```python
from build123d import *

# Parameters (mm, degrees)
PAD_DEPTH       = 10
POCKET_DEPTH    = 10.001
SKETCH002_W     = 1
SKETCH002_H     = 10
PAD001_DEPTH    = 7
SKETCH003_R     = 2
POCKET001_DEPTH = 5
FILLET_R        = 1


with BuildPart() as part:
    # Sketch → Pad (new body)
    with BuildSketch(Plane.XZ):
        with BuildLine():
            ThreePointArc((3.5, 3.5), (0, 6), (-3.5, 3.5))
            Line((-3.5, 3.5), (-3.5, 0))
            Line((-3.5, 0), (3.5, 0))
            Line((3.5, 0), (3.5, 3.5))
        make_face()
    extrude(amount=PAD_DEPTH)

    # Sketch001 (on Face6 of Pad) → Pocket (cut, through all)
    with BuildSketch(Plane.XZ.offset(10)):
        with BuildLine():
            ThreePointArc((2.5, 2.5), (0, 5), (-2.5, 2.5))
            Line((-2.5, 2.5), (-2.5, 0))
            Line((-2.5, 0), (2.5, 0))
            Line((2.5, 0), (2.5, 2.5))
        make_face()
    extrude(amount=-POCKET_DEPTH, mode=Mode.SUBTRACT)

    # Sketch002 (on Face3 of Pocket) → Pad001 (join)
    with BuildSketch(Plane(origin=(-3.5, 0, 0), x_dir=(0, 0, -1), z_dir=(-1, 0, 0))):
        with Locations((-0.5, 5)):
            Rectangle(SKETCH002_W, SKETCH002_H)
    extrude(amount=PAD001_DEPTH)

    # Sketch003 (on Face7 of Pad001) → Pocket001 (cut)
    with BuildSketch(Plane(origin=(0, 0, 1), x_dir=(-1, 0, 0), z_dir=(0, 0, 1))):
        with Locations((7, 5)):
            Circle(SKETCH003_R)
    extrude(amount=-POCKET001_DEPTH, mode=Mode.SUBTRACT)

    # Fillet
    fillet_edges = [part.edges().sort_by_distance(p)[0] for p in [
        (-10.5, -10, 0.5),
        (-10.5, 0, 0.5),
    ]]
    fillet(fillet_edges, radius=FILLET_R)


solid = part.part
```
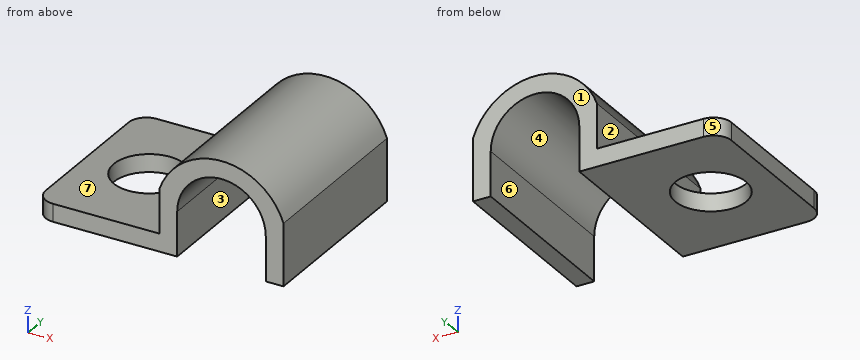
Source: CAD feature listing. Evaluate the final solid. Frame: model axes, mm. Face numbers are marked on the shaded views. A direction names the side the tool comes from. Coordinates: 2 decimals unless noted, no trailing zeros. Write each loop counter-clockwise with the first axis right and the second up, starting at its lowest first coordinate (ties: lowest second). Pieces come first, ordered by that corner, then holes. Notation, with made-up numbers: (86.25, 60.25) - (104.25, 60.25) arc R27 ccw to (104.25, 84.25) - close; hole circle Ø10 at (64, 77). An arc over 180 degrees is marked (long way). Answer as a JSON object with one key per item and string values.
Q1. Set-up query: the marked faces 1, 2 and 3. Return all of +Z, -Z, +X, -X, +Y, -Y with unobstructed straight access to the full face (end or side cutting, diameter ignored); none if empty.
Ans:
{"face 1": "+Z, -Z, +X, -X, +Y", "face 2": "+Z, -X, +Y, -Y", "face 3": "-Z, +Y, -Y"}
Q2. Section query B-B, the plane z = 1.8. Output: boundary loops of the cut face in (x, y), plus the area to 3 significant figures.
Ans:
{"outline": "(-3.5, -10) - (-2.5, -10) - (-2.5, 0) - (-3.5, 0) - close; (2.5, -10) - (3.5, -10) - (3.5, 0) - (2.5, 0) - close", "area": "20.0 mm2"}
Q3. Material intervals for line 1 (X direction, y = -5, z = 0.85); line 2 (X direction, y = -6.5, z = 2.3); line 3 (X direction, y = -5.5, z = 0.55), sorted ascending. Write a range as [from, to].
Ans:
{"line 1": "x = [-10.5, -9], [-5, -2.5], [2.5, 3.5]", "line 2": "x = [-3.5, -2.5], [2.5, 3.5]", "line 3": "x = [-10.5, -8.94], [-5.06, -2.5], [2.5, 3.5]"}
Q4. Section query A-A, the plane x = -7. Output: boundary loops of the cut face in (y, z), plus the area to 3 significant figures.
Ans:
{"outline": "(-10, 0) - (-7, 0) - (-7, 1) - (-10, 1) - close; (-3, 0) - (0, 0) - (0, 1) - (-3, 1) - close", "area": "6.00 mm2"}
Q5. First-contact query: pin 1 Ø1.5 at (x, z) = (-7.5, 2.5) entering from -Y; pin 2 Ø5.5 at (x, y) = (-8.5, -3) entering from +Z; pin 3 Ø1 at (y, z) = (-4.5, 5) entering from +X. Flat tips, straight axial feed; report the tip coordinate or a pass-through.
Ans:
{"pin 1": "passes through", "pin 2": "stops at z = 1", "pin 3": "stops at x = 2.97"}
Q6. Draft query along X for the marked faces 4, 5, 6 and 7. Return one class per face: released by +X, released by -X, zero draft, split by the parting line, or undercut.
Ans:
{"face 4": "undercut", "face 5": "released by -X", "face 6": "undercut", "face 7": "zero draft"}
Q7. Section query C-C, the plane y = -5. Output: boundary loops of the cut face in (x, z).
Ans:
{"outline": "(-10.5, 0) - (-9, 0) - (-9, 1) - (-10.5, 1) - close; (-5, 0) - (-2.5, 0) - (-2.5, 2.5) arc R2.5 cw to (2.5, 2.5) - (2.5, 0) - (3.5, 0) - (3.5, 3.5) arc R3.7 ccw to (-3.5, 3.5) - (-3.5, 1) - (-5, 1) - close"}
Q8. Section query D-D, the plane y = -7.75. Output: boundary loops of the cut face in (x, z).
Ans:
{"outline": "(-10.5, 0) - (-2.5, 0) - (-2.5, 2.5) arc R2.5 cw to (2.5, 2.5) - (2.5, 0) - (3.5, 0) - (3.5, 3.5) arc R3.7 ccw to (-3.5, 3.5) - (-3.5, 1) - (-10.5, 1) - close"}
